The drawing under review shows one solid part. Ordinate dimensions are in mm from its lowest x, y, z. A direction names the side the tool comes from. Coordinates: 2 decimals unless noted, no trailing zeros. Write each loop counter-clockwise with the first axis right and the second up, starting at its lowest first coordinate (ties: lowest second). Pieces come first, ordered by that corner, then holes.
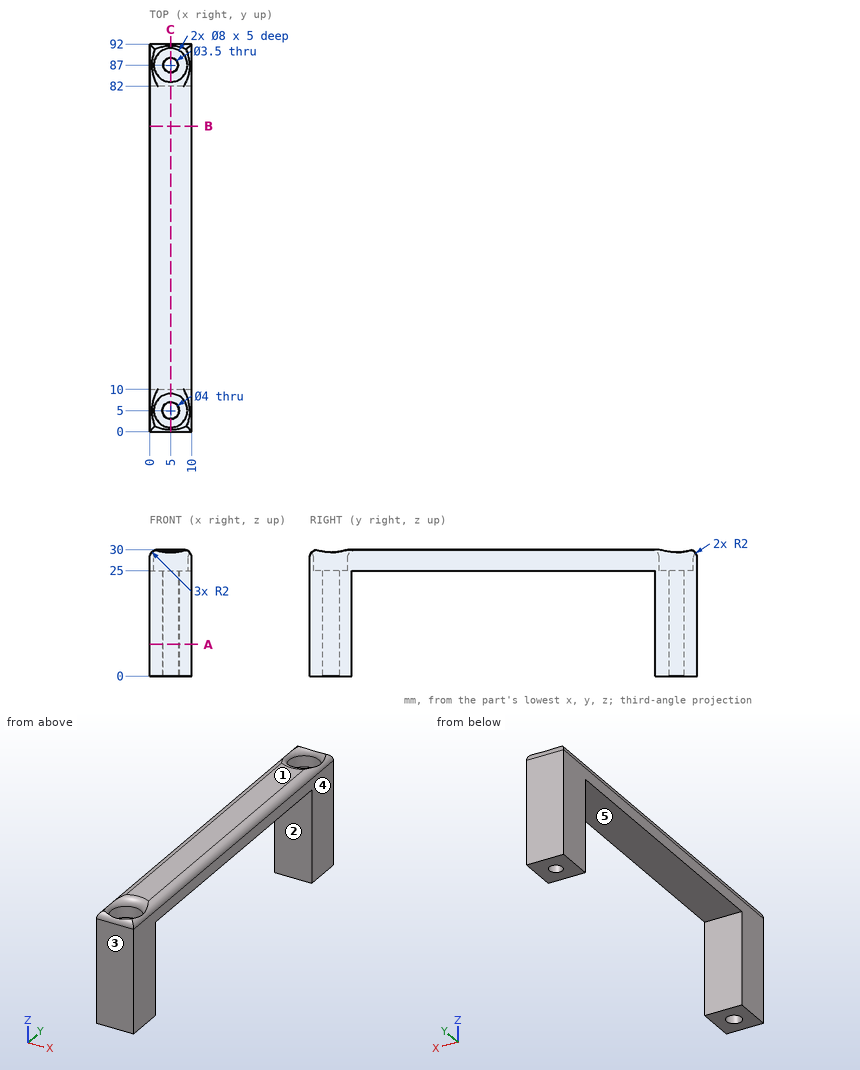
Q1. Add section A-A (z = 7.5). State the section outline as (x, y) points, then the cut area to 3 significant figures.
Ans:
outline: (0, 0) - (10, 0) - (10, 10) - (0, 10) - close; (0, 82) - (10, 82) - (10, 92) - (0, 92) - close; hole circle Ø4 at (5, 5); hole circle Ø3.5 at (5, 87)
area: 178 mm2
Q2. Add section B-B (y = 72.5). State the section outline as (x, z) points, then the cut area to 3 significant figures.
Ans:
outline: (0, 25) - (10, 25) - (10, 28) arc R2 ccw to (8, 30) - (2, 30) arc R2 ccw to (0, 28) - close
area: 48.3 mm2
Q3. For probe 1 along Y at (x, z) = (5, 25.75); probe 2 along Y at (x, z) = (5, 17); probe 3 along Y at (x, z) = (8.75, 4.5), list the stretches that pass through material, from the lowest coordinate up.
Ans:
probe 1: y = 0 to 1, 9 to 83, 91 to 92
probe 2: y = 0 to 3, 7 to 10, 82 to 85.25, 88.75 to 92
probe 3: y = 0 to 10, 82 to 92
Q4. Clearance check with a flat-ended pin moving along its axis: pin 1 Ø2.5 at (x, y) = (6, 4.5) entering from +Z. State where the tip first meets the part, or that it passes through.
Ans:
pin 1: stops at z = 25
Q5. Add section C-C (x = 5). Give the number of separate pieces and of enclosed holes in the cut face, then the cut area to 3 significant figures.
Ans:
separate pieces: 3
enclosed holes: 0
area: 689 mm2
Q6. Draft analysis for pull direction Y (two halves, no side actions). For the marked faces 3, 4 and 5, state which applies: +Y half, -Y half, draft (parallel to the pull), parting line (faces both ways), or undercut.
Ans:
face 3: -Y half
face 4: draft
face 5: undercut
Q7. Tool access review of the marked faces 1 and 2: name each direction out of +Z, -Z, +X, -X, +Y, -Y from which nothing blocks a thin tool from reaching the whole face with its end or side.
Ans:
face 1: +Z, +X, -X, +Y, -Y
face 2: -Z, +X, -X
